Here's how the part is built. I have some questions about the finished solid (model axes, mm). Face numbers are marked on the shaded views. A direction names the side the tool comes from. Round coordinates to 2 decimals unless told otherwise and drop trailing zeros. Order: outer loops, then holes, each group sorted by start corner. A loop starts at its lowest first (then second) coordinate and runs counter-clockwise, first axis right, second up. Notation, with made-up numbers: (-34.5, 79.5) -> (-1.5, 79.5) arc R25 cw to (-1.5, 104.5) -> close; hole circle Ø2 at (-29, 26). An arc over 180 degrees is marked (long way). Use a Markdown table: item, result. Add a question column.
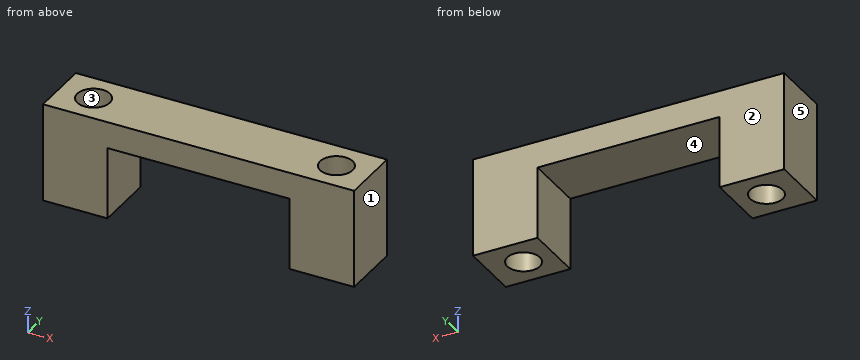
Autodesk Fusion 360 part; units mm, degrees
sketch "Sketch1" plane through (0, 0, 0) normal (0, 0, 1) x (1, 0, 0)
  line L0 (20.5, -4) -> (-20.5, -4)
  line L1 (-20.5, -4) -> (-20.5, 4)
  line L2 (-20.5, 4) -> (20.5, 4)
  line L3 (20.5, 4) -> (20.5, -4)
  line L4 (20.5, -4) -> (-20.5, 4) construction
  line L5 (-20.5, -4) -> (20.5, 4) construction
  line L6 (-16, 0) -> (16, 0) construction
  circle A0 centre (-16, 0) radius 2.15
  circle A1 centre (16, 0) radius 2.15
  dimension "d1" = 8
  dimension "d2" = 41
  dimension "d3" = 32
  dimension "d4" = 4.3
  dimension "d5" = 4.3
extrude "Extrude1" add sketch "Sketch1" along normal blind 13
sketch "Sketch3" plane through (0, 0, 0) normal (0, 0, -1) x (1, 0, 0)
  circle A0 centre (16, 0) radius 2.15
  circle A1 centre (-16, 0) radius 2.15
  line L0 (-20.5, -4) -> (20.5, -4)
  line L1 (20.5, -4) -> (20.5, 4)
  line L2 (20.5, 4) -> (-20.5, 4)
  line L3 (-20.5, 4) -> (-20.5, -4)
  line L4 (12, -4) -> (-12, -4)
  line L5 (-12, -4) -> (-12, 4)
  line L6 (-12, 4) -> (12, 4)
  line L7 (12, 4) -> (12, -4)
  line L8 (12, -4) -> (-12, 4) construction
  line L9 (-12, -4) -> (12, 4) construction
  dimension "d9" = 24
extrude "Extrude2" cut sketch "Sketch3" against normal blind 9.5 contours L0 L2 L4 L5 L6 L7
(1) I want a section at D-D on z = 11. List the corners of the cut face in (x, y) for me.
(2) I want a section at C-C on y = 0. List the corners of the cut face in (x, z) for me.
(3) If we mould it in two halves opening along X, with no side actions, what happens to the marked faces 1, 2 and 3? For each: pulls with the +X half, pulls with the -X half, needs draft (parallel to the pull), parting line crosses it, or undercut.
(4) I want a section at A-A on z = 6.25. List the corners of the cut face in (x, y) for me.
(5) Please list where these lines run through material, in increasing order: probe 1 along Y at (x, z) = (16, 9); probe 2 along X at (y, z) = (3.5, 4.25); probe 3 along X at (y, z) = (-1.75, 11). Write a range as from..to.
(6) On a 3-axis mill with a long thin cutter (end or side, diameter ignored), from which of +Z, -Z, +X, -X, +Y, -Y can I reach the whole of each face in a straight line? I mean the marked faces 4 and 5. Say none if no direction works.
(7) I want a section at B-B on x = 16. List the corners of the cut face in (y, z) for me.
(8) I'm going to push a flat-ended pin straight in: P1, Ø4, axis at x = -2, y = -2, coming from the -Z side. Where does the tip first touch, or does it pass through?
Output:
| question | item | result |
|---|---|---|
| 1 | outline | (-20.5, -4) -> (20.5, -4) -> (20.5, 4) -> (-20.5, 4) -> close; hole circle Ø4.3 at (-16, 0); hole circle Ø4.3 at (16, 0) |
| 2 | outline | (-20.5, 0) -> (-18.15, 0) -> (-18.15, 13) -> (-20.5, 13) -> close; (-13.85, 0) -> (-12, 0) -> (-12, 9.5) -> (12, 9.5) -> (12, 0) -> (13.85, 0) -> (13.85, 13) -> (-13.85, 13) -> close; (18.15, 0) -> (20.5, 0) -> (20.5, 13) -> (18.15, 13) -> close |
| 3 | face 1 | pulls with the +X half |
| 3 | face 2 | needs draft |
| 3 | face 3 | undercut |
| 4 | outline | (-20.5, -4) -> (-12, -4) -> (-12, 4) -> (-20.5, 4) -> close; (12, -4) -> (20.5, -4) -> (20.5, 4) -> (12, 4) -> close; hole circle Ø4.3 at (-16, 0); hole circle Ø4.3 at (16, 0) |
| 5 | probe 1 | -4..-2.15, 2.15..4 |
| 5 | probe 2 | -20.5..-12, 12..20.5 |
| 5 | probe 3 | -20.5..-17.25, -14.75..14.75, 17.25..20.5 |
| 6 | face 4 | -Z, +Y, -Y |
| 6 | face 5 | +Z, -Z, -X, +Y, -Y |
| 7 | outline | (-4, 0) -> (-2.15, 0) -> (-2.15, 13) -> (-4, 13) -> close; (2.15, 0) -> (4, 0) -> (4, 13) -> (2.15, 13) -> close |
| 8 | P1 | z = 9.5 |
